from build123d import *

# Parameters (mm, degrees)
SKETCH2_W           = 213.36
SKETCH2_H           = 213.36
SKETCH2_R           = 93.98
BOSS_EXTRUDE1_DEPTH = 50.8
SKETCH4_W           = 431.498092941
SKETCH4_H           = 427.351859682
CUT_EXTRUDE1_DEPTH  = 106.68
FILLET1_R           = 2.54
SKETCH6_W           = 213.36
SKETCH6_H           = 50.8
BOSS_EXTRUDE3_DEPTH = 76.2


with BuildPart() as part:
    # Sketch2 → Boss-Extrude1 (new body)
    with BuildSketch(Plane.XY.offset(50.8)):
        Rectangle(SKETCH2_W, SKETCH2_H)
        Circle(SKETCH2_R, mode=Mode.SUBTRACT)
    extrude(amount=-BOSS_EXTRUDE1_DEPTH)

    # Cut-Loft1: read off the stored shape, not the designer's step
    # Cut-Loft1: loft between two sections, ruled curve by curve
    cut_loft1_from = [
        Edge.make_bspline([(-5.225836659, 98.922061398, 0), (-203.069959455, 88.47038808, 0), (-192.618286137, -109.373734716, 0), (5.225836659, -98.922061398, 0), (203.069959455, -88.47038808, 0), (192.618286137, 109.373734716, 0), (-5.225836659, 98.922061398, 0)], [0, 0, 0, 0, 0.5, 0.5, 0.5, 1, 1, 1, 1], 3, [1, 0.333333333, 0.333333333, 1, 0.333333333, 0.333333333, 1]),
    ]
    cut_loft1_to = [
        Edge.make_bspline([(82.069205503, 45.791766816, 50.8), (-9.514328128, 209.930177822, 50.8), (-173.652739134, 118.34664419, 50.8), (-82.069205503, -45.791766816, 50.8), (9.514328128, -209.930177822, 50.8), (173.652739134, -118.34664419, 50.8), (82.069205503, 45.791766816, 50.8)], [0, 0, 0, 0, 0.5, 0.5, 0.5, 1, 1, 1, 1], 3, [1, 0.333333333, 0.333333333, 1, 0.333333333, 0.333333333, 1]),
    ]
    cut_loft1 = Solid(Shell([*[Face.make_surface_from_curves(cut_loft1_from[k], cut_loft1_to[k]) for k in range(1)], Face(Wire(cut_loft1_from)), Face(Wire(cut_loft1_to))]))
    add(cut_loft1, mode=Mode.SUBTRACT)

    # Sketch4 → Cut-Extrude1 (cut)
    with BuildSketch(Plane(origin=(0, 106.68, 0), x_dir=(1, 0, 0), z_dir=(0, 1, 0))):
        with Locations((-43.743226098, -53.764043901)):
            Rectangle(SKETCH4_W, SKETCH4_H)
    extrude(amount=-CUT_EXTRUDE1_DEPTH, mode=Mode.SUBTRACT)

    # Fillet1
    fillet1_edges = [part.edges().sort_by_distance(p)[0] for p in [
        (93.98, 0, 27.785112978),
        (-93.98, 0, 27.785112678),
    ]]
    fillet(fillet1_edges, radius=FILLET1_R)

    # Sketch6 → Boss-Extrude3 (add)
    with BuildSketch(Plane(origin=(0, -106.68, 0), x_dir=(-1, 0, 0), z_dir=(0, -1, 0))):
        with Locations((0, -25.4)):
            Rectangle(SKETCH6_W, SKETCH6_H)
    extrude(amount=BOSS_EXTRUDE3_DEPTH)


solid = part.part
Read the model definition and answer for the solid it produces. Units are mm, in the model's axes. Coordinates: 2 decimals unless noted, no trailing zeros. Loops run counter-clockwise (first coordinate to the right, second up) from the corner with the lowest first, then second, coordinate; pieces in that order, holes last. Notation, with made-up numbers: (63, 18) - (117, 18) arc R37 cw to (117, 54) - close; hole circle Ø4 at (66.5, -14.75). An arc over 180 degrees is marked (long way). Answer in a Markdown table with one row per item.
Q1. The mould has two halves that part along X. Classify faces 1 (the cylindrical face through (-2.03, -93.96, 28.11)), 2 (the flat face through (106.68, -90, 26)), 3 (the flat face through (1, -131, 0)): pulls with the +X half, pulls with the -X half, needs draft (parallel to the pull), parting line crosses it, or undercut.
Here are the results:
| item | result |
|---|---|
| face 1 | undercut |
| face 2 | pulls with the +X half |
| face 3 | needs draft |
Q2. Given P1, Ø12, axis at x = 38.5, z = 8, coming from the +Y side; P2, Ø8, axis at x = -13, y = -158.5, coming from the -Z side; P3, Ø1.5, axis at x = 28.5, z = 23.5, coming from the +Y side; P4, Ø6, axis at x = 57, z = 45.5, coming from the +Y side, each flat-ended and moving along its own axis, determine where each tip first touches the part or whether it passes through.
Here are the results:
| item | result |
|---|---|
| P1 | stops at y = -82.78 |
| P2 | stops at z = 0 |
| P3 | stops at y = -89.31 |
| P4 | stops at y = -72.33 |
Q3. Straight lines are drawn through the part: line 1 along X through (y, z) = (-19.5, 13); line 2 along X through (y, z) = (-73.5, 13); line 3 along Y through (x, z) = (-71, 42.5). For each, find the intervals that lie inside material, in ascending order. Write a range as [from, to].
Here are the results:
| item | result |
|---|---|
| line 1 | x = [-106.68, -91.93], [91.93, 106.68] |
| line 2 | x = [-106.68, -58.57], [58.57, 106.68] |
| line 3 | y = [-182.88, -61.57] |
Q4. Find section A-A on z = 13. Write down the section's boundary in (x, y).
Here are the results:
| item | result |
|---|---|
| outline | (-106.68, -182.88) - (106.68, -182.88) - (106.68, 0) - (96.49, 0) arc R2.54 ccw to (93.95, -2.47) arc R93.98 cw to (-93.95, -2.47) arc R2.54 ccw to (-96.49, 0) - (-106.68, 0) - close |
